The listing builds one solid part. Answer for the finished solid, in the listing's coordinates (mm). Face numbers are marked on the shaded views. A direction names the side the tool comes from. Round coordinates to 2 decimals unless told otherwise and drop trailing zeros. Write each loop counter-clockwise with the first axis right and the second up, starting at its lowest first coordinate (ties: lowest second). Pieces come first, ordered by that corner, then holes. Notation, with made-up numbers: (-10, 71) - (-4, 71) arc R8 cw to (-4, 83) - close; hole circle Ø5 at (73, 17.25). An arc over 180 degrees is marked (long way). Return JSON: item names as keys, results as strings. Group by question number.
(1) Which of the six approach directions +Z, -Z, +X, -X, +Y, -Y give full straight-line access (tool end or side, diameter ignored) to the marked faces 5, 6, 7 and 8?
(2) Determine the mould class of the marked faces 1, 2, 3 and 4 for opening direction Y: +Y half, -Y half, draft (parallel to the pull), parting line (faces both ways), or undercut.
(3) Section B-B, the plane y = 17.5 is taken. Write down the section's boundary in (x, z), then the cut area to 3 significant figures.
(4) Each of these flat-tipped pins is pushed along its axis until it touches: pin 1 (1.8 mm diameter, centred on x = 3.5, y = 3.5, fed in from -Z); pin 2 (2.5 mm diameter, centred on x = -4, z = 0.5, fed in from +Y); pin 3 (4 mm diameter, centred on x = 4.5, y = 3.5, fed in from +Z). Where does it stop, or does it pass through?
(5) Find the intervals of material crossed by line 1 along Z through (x, y) = (1.5, 4); line 2 along Y through (x, z) = (3.75, 1.45); line 3 along Y through (x, z) = (2.75, -0.6), in increasing order. Write a range as [from, to].
(6) Section A-A, the plane y = 27 is taken. Write down the section's boundary in (x, z).
```python
from build123d import *
from build123d.topology import SkipClean

# Parameters (mm, degrees)
SKETCH1_R           = 2.35
BOSS_EXTRUDE1_DEPTH = 6
SKETCH2_R           = 2.35
BOSS_EXTRUDE2_DEPTH = 16
BOSS_EXTRUDE3_START = 22
SKETCH1_2_R         = 2.35
BOSS_EXTRUDE3_DEPTH = 14
BOSS_EXTRUDE4_START = 30
SKETCH2_2_R         = 2.35
BOSS_EXTRUDE4_DEPTH = 20.5
CHAMFER1_SIZE       = 3


with BuildPart() as part:
    # Sketch1 → Boss-Extrude1 (new body)
    with BuildSketch(Plane(origin=(0, 0, 0), x_dir=(1, 0, 0), z_dir=(0, 1, 0))):
        with BuildLine():
            Line((-5.35, -1.5), (-1.809005252, -1.5))
            ThreePointArc((-1.809005252, -1.5), (-2.35, 0), (-1.809005252, 1.5))
            Line((-1.809005252, 1.5), (-5.35, 1.5))
            Line((-5.35, 1.5), (-5.35, -1.5))
        make_face()
        Circle(SKETCH1_R)
        with BuildLine():
            ThreePointArc((2.35, 0), (2.210617826, -0.797288423), (1.809005252, -1.5))
            Line((1.809005252, -1.5), (5.35, -1.5))
            Line((5.35, -1.5), (5.35, 1.5))
            Line((5.35, 1.5), (1.809005252, 1.5))
            ThreePointArc((1.809005252, 1.5), (2.210617826, 0.797288423), (2.35, 0))
        make_face()
    extrude(amount=BOSS_EXTRUDE1_DEPTH)

    # Sketch2 → Boss-Extrude2 (add)
    with BuildSketch(Plane(origin=(0, 6, 0), x_dir=(1, 0, 0), z_dir=(0, 1, 0))):
        with Locations(Location((0, 0, 0), (0, 0, 39.665012908))):
            Circle(SKETCH2_R)
    extrude(amount=BOSS_EXTRUDE2_DEPTH)

    # Sketch1<2> → Boss-Extrude3 (add)
    with BuildSketch(Plane(origin=(0, 0, 0), x_dir=(1, 0, 0), z_dir=(0, 1, 0)).offset(BOSS_EXTRUDE3_START)):
        with BuildLine():
            Line((-5.35, -1.5), (-1.809005252, -1.5))
            ThreePointArc((-1.809005252, -1.5), (-2.35, 0), (-1.809005252, 1.5))
            Line((-1.809005252, 1.5), (-5.35, 1.5))
            Line((-5.35, 1.5), (-5.35, -1.5))
        make_face()
        with Locations(Location((0, 0, 0), (0, 0, 39.665012908))):
            Circle(SKETCH1_2_R)
        with BuildLine():
            ThreePointArc((2.35, 0), (2.210617826, -0.797288423), (1.809005252, -1.5))
            Line((1.809005252, -1.5), (5.35, -1.5))
            Line((5.35, -1.5), (5.35, 1.5))
            Line((5.35, 1.5), (1.809005252, 1.5))
            ThreePointArc((1.809005252, 1.5), (2.210617826, 0.797288423), (2.35, 0))
        make_face()
    extrude(amount=BOSS_EXTRUDE3_DEPTH)

    # Sketch2<2> → Boss-Extrude4 (add)
    with SkipClean():  # the faces are left unmerged after this step: merging them gives an invalid solid
        with BuildSketch(Plane(origin=(0, 6, 0), x_dir=(1, 0, 0), z_dir=(0, 1, 0)).offset(BOSS_EXTRUDE4_START)):
            with Locations(Location((0, 0, 0), (0, 0, 39.665012908))):
                Circle(SKETCH2_2_R)
        extrude(amount=BOSS_EXTRUDE4_DEPTH)

    # Chamfer1
    # the kernel refuses this chamfer: 3 mm, written as the material it adds along each edge
    with BuildSketch(Plane(origin=(0, 22, 0), x_dir=(-0.9999950652018471, 0, 0.003141587489430323), z_dir=(-0.003141587489430323, 0, -0.9999950652018471))) as chamfer1_piece_1_section:
        Polygon((2.35, -CHAMFER1_SIZE), (2.35 + CHAMFER1_SIZE, 0), (2.35, 0), align=None)
    chamfer1_piece_1 = revolve(axis=Axis((0, 22, 0), (0, 1, 0)), revolution_arc=359.64, mode=Mode.PRIVATE)
    chamfer1_piece_1 = split(chamfer1_piece_1, bisect_by=Plane(origin=(-3.19448265, 21.00212183, 1.5), z_dir=(0, 0, -1)), keep=Keep.TOP, mode=Mode.PRIVATE)
    chamfer1_piece_1 = split(chamfer1_piece_1, bisect_by=Plane(origin=(-3.19448265, 21.00212183, -1.5), z_dir=(0, 0, 1)), keep=Keep.TOP, mode=Mode.PRIVATE)
    chamfer1_piece_1 = split(chamfer1_piece_1, bisect_by=Plane(origin=(5.35, 21.00212183, 0.771950274), z_dir=(-1, 0, 0)), keep=Keep.TOP, mode=Mode.PRIVATE)
    add(chamfer1_piece_1)
    with BuildSketch(Plane(origin=(0, 22, 0), x_dir=(0.9999950652018581, 0, -0.0031415874858800653), z_dir=(0.0031415874858800653, 0, 0.9999950652018581))) as chamfer1_piece_2_section:
        Polygon((2.35, -CHAMFER1_SIZE), (2.35 + CHAMFER1_SIZE, 0), (2.35, 0), align=None)
    chamfer1_piece_2 = revolve(axis=Axis((0, 22, 0), (0, 1, 0)), revolution_arc=359.64, mode=Mode.PRIVATE)
    chamfer1_piece_2 = split(chamfer1_piece_2, bisect_by=Plane(origin=(3.19448265, 21.00212183, 1.5), z_dir=(0, 0, -1)), keep=Keep.TOP, mode=Mode.PRIVATE)
    chamfer1_piece_2 = split(chamfer1_piece_2, bisect_by=Plane(origin=(3.19448265, 21.00212183, -1.5), z_dir=(0, 0, 1)), keep=Keep.TOP, mode=Mode.PRIVATE)
    chamfer1_piece_2 = split(chamfer1_piece_2, bisect_by=Plane(origin=(-5.35, 21.00212183, -0.771950274), z_dir=(1, 0, 0)), keep=Keep.TOP, mode=Mode.PRIVATE)
    add(chamfer1_piece_2)


solid = part.part
```
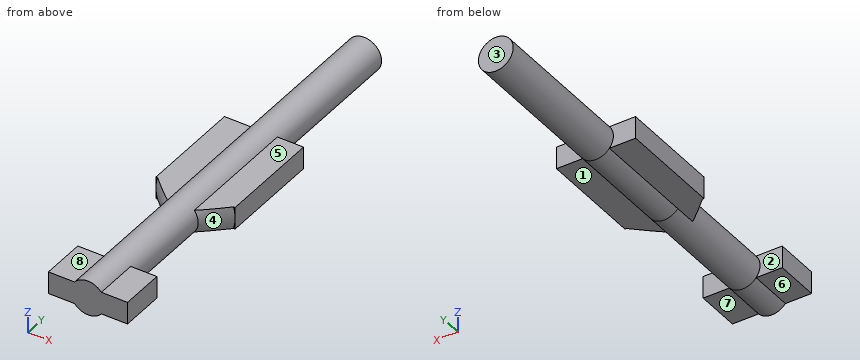
Working result:
{
 "1": {"face 5": "+Z, +X, +Y, -Y", "face 6": "-Z, -X, +Y, -Y", "face 7": "-Z, +X, +Y, -Y", "face 8": "+Z, -X, +Y, -Y"},
 "2": {"face 1": "draft", "face 2": "undercut", "face 3": "+Y half", "face 4": "undercut"},
 "3": {"outline": "circle Ø4.7 at (0, 0)", "area": "17.3 mm^2"},
 "4": {"pin 1": "stops at z = -1.5", "pin 2": "stops at y = 36", "pin 3": "stops at z = 1.5"},
 "5": {"line 1": "z = [-1.81, 1.81]", "line 2": "y = [0, 6], [20.67, 36]", "line 3": "y = [0, 6], [19.46, 36]"},
 "6": {"outline": "(-5.35, -1.5) - (-1.81, -1.5) arc R2.35 ccw to (1.81, -1.5) - (5.35, -1.5) - (5.35, 1.5) - (1.81, 1.5) arc R2.35 ccw to (-1.81, 1.5) - (-5.35, 1.5) - close"}
}
